```python
from build123d import *

# Parameters (mm, degrees)
SKETCH_1_W          = 27
SKETCH_1_H          = 20.5
EXTRUDE_1_DEPTH     = 15
SKETCH_2_W          = 0.8
SKETCH_2_H          = 4.8
EXTRUDE_2_DEPTH     = 9
CHAMFER_1_SIZE      = 1
SKETCH_3_W          = 31
SKETCH_3_H          = 24
EXTRUDE_3_DEPTH     = 3
CUT_EXTRUDE_1_DEPTH = 17
SKETCH_5_W          = 2
SKETCH_5_H          = 4
EXTRUDE_4_DEPTH     = 15
CHAMFER_2_SIZE      = 0.8


with BuildPart() as part:
    # Эскиз1 → Бобышка-Вытянуть1 (new body)
    with BuildSketch(Plane(origin=(0, 0, 0), x_dir=(1, 0, 0), z_dir=(0, 1, 0))):
        Rectangle(SKETCH_1_W, SKETCH_1_H)
    extrude(amount=EXTRUDE_1_DEPTH)

    # Эскиз2 → Бобышка-Вытянуть2 (add)
    with BuildSketch(Plane.XZ):
        with Locations((0, 3)):
            Rectangle(SKETCH_2_W, SKETCH_2_H)
        with Locations((-7, -3)):
            Rectangle(SKETCH_2_W, SKETCH_2_H)
        with Locations((7, -3)):
            Rectangle(SKETCH_2_W, SKETCH_2_H)
    extrude(amount=EXTRUDE_2_DEPTH)

    # Фаска1
    chamfer_1_edges = [part.edges().sort_by_distance(p)[0] for p in [
        (-7, -9, -0.6),
        (-7, -9, -5.4),
        (0, -9, 5.4),
        (0, -9, 0.6),
        (7, -9, -0.6),
        (7, -9, -5.4),
    ]]
    chamfer(chamfer_1_edges, length=CHAMFER_1_SIZE)

    # Эскиз3 → Бобышка-Вытянуть3 (add)
    with BuildSketch(Plane(origin=(0, 15, 0), x_dir=(1, 0, 0), z_dir=(0, 1, 0))):
        Rectangle(SKETCH_3_W, SKETCH_3_H)
    extrude(amount=EXTRUDE_3_DEPTH)

    # Эскиз4 → Вырез-Вытянуть1 (cut)
    with BuildSketch(Plane(origin=(0, 18, 0), x_dir=(1, 0, 0), z_dir=(0, 1, 0))):
        Polygon((12, -3), (7, -8), (-7, -8), (-12, -3), (-12, 8), (12, 8), align=None)
    extrude(amount=-CUT_EXTRUDE_1_DEPTH, mode=Mode.SUBTRACT)

    # Эскиз5 → Бобышка-Вытянуть4 (add)
    with BuildSketch(Plane(origin=(0, 1, 0), x_dir=(1, 0, 0), z_dir=(0, 1, 0))):
        with Locations((7, 2)):
            Rectangle(SKETCH_5_W, SKETCH_5_H)
        with Locations((0, -2)):
            Rectangle(SKETCH_5_W, SKETCH_5_H)
        with Locations((-7, 2)):
            Rectangle(SKETCH_5_W, SKETCH_5_H)
    extrude(amount=EXTRUDE_4_DEPTH)

    # Фаска2
    chamfer_2_edges = [part.edges().sort_by_distance(p)[0] for p in [
        (-1, 16, 2),
        (0, 16, 4),
        (1, 16, 2),
        (0, 16, 0),
        (6, 16, -2),
        (7, 16, 0),
        (8, 16, -2),
        (7, 16, -4),
        (-7, 16, -4),
        (-8, 16, -2),
        (-7, 16, 0),
        (-6, 16, -2),
    ]]
    chamfer(chamfer_2_edges, length=CHAMFER_2_SIZE)


solid = part.part
```
The model under review builds one solid part; all positions refer to its coordinate system, in mm. A direction names the side the tool comes from. Give positions to 0.01 mm unless a question says otherwise; leave off trailing zeros. Loops run counter-clockwise (first coordinate to the right, second up) from the corner with the lowest first, then second, coordinate; pieces in that order, holes last. Notation, with made-up numbers: (-4, 29.25) - (14, 29.25) arc R21 ccw to (14, 63.25) - close; hole circle Ø9 at (37.5, 23.5). An arc over 180 degrees is marked (long way). Answer as a JSON object with one key per item and string values.
Q1. To check wall thickness, follow line 1 along X through (y, z) = (9, 1); line 2 along Z through (x, y) = (-6.5, 16.75); line 3 along Z through (x, y) = (9, 6.5). State the ranges of each line that lie inside material, in increasing order.
Worked out:
{"line 1": "x = -13.5 to -12, -1 to 1, 12 to 13.5", "line 2": "z = -12 to -8, 8 to 12", "line 3": "z = -10.25 to -8, 6 to 10.25"}
Q2. Add section B-B on y = -1.25. State the section outline as (x, z) points.
Worked out:
{"outline": "(-7.4, -5.4) - (-6.6, -5.4) - (-6.6, -0.6) - (-7.4, -0.6) - close; (-0.4, 0.6) - (0.4, 0.6) - (0.4, 5.4) - (-0.4, 5.4) - close; (6.6, -5.4) - (7.4, -5.4) - (7.4, -0.6) - (6.6, -0.6) - close"}
Q3. Add section C-C on z = -7.5. State the section outline as (x, y) points.
Worked out:
{"outline": "(-15.5, 15) - (-13.5, 15) - (-13.5, 0) - (13.5, 0) - (13.5, 15) - (15.5, 15) - (15.5, 18) - (12, 18) - (12, 1) - (-12, 1) - (-12, 18) - (-15.5, 18) - close"}
Q4. Mouldability with a two-part tool opening along X and no side actions: class faces 5 (the flat face through (0, -8.5, 1.1)), 6 (the flat face through (0, 10, -8)) as +X half, -X half, draft (parallel to the pull), parting line (faces both ways), or undercut.
Worked out:
{"face 5": "draft", "face 6": "undercut"}
Q5. Add section A-A on y = 4.25. State the section outline as (x, z) points, plus the area to 4 significant figures.
Worked out:
{"outline": "(-13.5, -10.25) - (13.5, -10.25) - (13.5, 10.25) - (-13.5, 10.25) - close; (-8, -4) - (-6, -4) - (-6, 0) - (-8, 0) - close; (-1, 0) - (1, 0) - (1, 4) - (-1, 4) - close; (6, -4) - (8, -4) - (8, 0) - (6, 0) - close; hole (-12, -8) - (12, -8) - (12, 3) - (7, 8) - (-7, 8) - (-12, 3) - close", "area": "218.5 mm^2"}
Q6. For faces 1 (the flat face through (-6.6, -4, -3)), 2 (the flat face through (7, -9, -3)), 3 (the flat face through (7, -4, -0.6)), 4 (the flat face through (8, 8, -2)), list the 3-axis set-ups (+Z, -Z, +X, -X, +Y, -Y) from which the entire face can be reached by the end or side of a thin tool; tool diameter is ignored.
Worked out:
{"face 1": "+Z, -Z, -Y", "face 2": "+Z, -Z, +X, -X, -Y", "face 3": "+Z, +X, -X, -Y", "face 4": "+Y"}
Q7. Insertion check: pin 1 (1.6 mm diameter, centred on x = 0, y = 6, fed in from -Z); pin 2 (2 mm diameter, centred on x = -0.5, z = -1, fed in from -Y); pin 3 (0.9 mm diameter, centred on x = -7, y = -5.5, fed in from -Z). Each pin has a flat end and moves straight along its axis. Give the tip position at first contact, or say it passes through.
Worked out:
{"pin 1": "stops at z = -10.25", "pin 2": "stops at y = 0", "pin 3": "stops at z = -5.4"}
Q8. Add section D-D on x = -12.5. State the section outline as (y, z) points, plus the area to 4 significant figures.
Worked out:
{"outline": "(0, -10.25) - (15, -10.25) - (15, -12) - (18, -12) - (18, 12) - (15, 12) - (15, 10.25) - (0, 10.25) - close", "area": "379.5 mm^2"}
